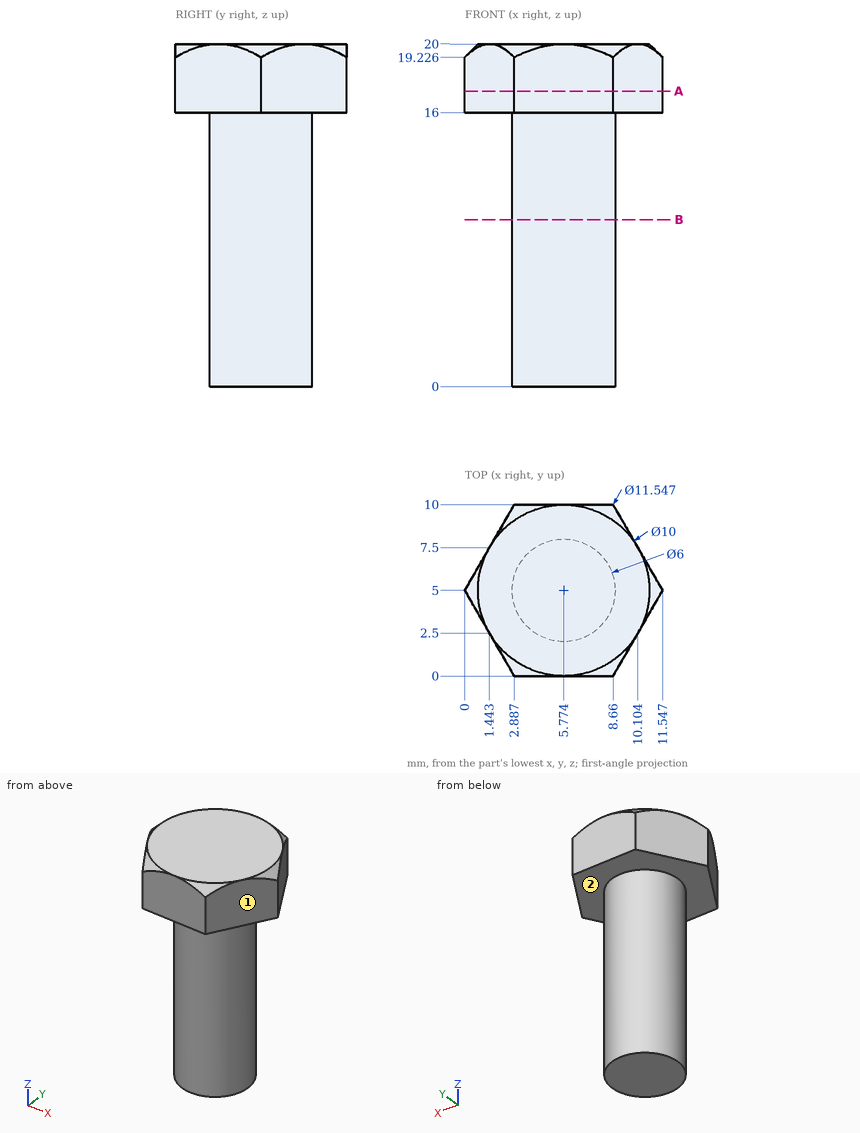
Here's the drawing with two shaded views (mm, measured from the low corner). I have some questions. A direction names the side the tool comes from. Coordinates: 2 decimals unless noted, no trailing zeros. Order: outer loops, then holes, each group sorted by start corner. A loop starts at its lowest first (then second) coordinate and runs counter-clockwise, first axis right, second up.
Q1. Suppose I cut it at B-B on z = 9.75. Please give me the cut outline in (x, y).
Q2. Suppose I cut it at A-A on z = 17.25. Please give me the cut outline in (x, y).
Q3. Will these pins go through, and if not, where does the flat tip stop? pin 1 (1 mm diameter, centred on x = 5.5, z = 4, fed in from +Y); pin 2 (6 mm diameter, centred on y = 1.5, z = 11.5, fed in from -X) (1 decimal); pin 3 (4 mm diameter, centred on y = 9, z = 16.5, fed in from +X).
Q4. Which directions (+Z, -Z, +X, -X, +Y, -Y) give clear straight access to the entire face, cutting with the end or side of a thin tool? Please do the marked faces 1 and 2.
Q5. Please list where these lines run through material, in increasing order: L1, parallel to Z at x = 1.5, y = 4.75; L2, parallel to X at y = 4.5, z = 2 (1 decimal); L3, parallel to Y at x = 5.25, z = 2.5 (1 decimal).
Answer:
1. outline: circle Ø6 at (5.77, 5)
2. outline: (0, 5) - (2.89, 0) - (8.66, 0) - (11.55, 5) - (8.66, 10) - (2.89, 10) - close
3. pin 1: stops at y = 8
3. pin 2: stops at x = 2.8
3. pin 3: stops at x = 10.39
4. face 1: +Z, -Z, +X, -Y
4. face 2: -Z
5. L1: z = 16 to 20
5. L2: x = 2.8 to 8.7
5. L3: y = 2 to 8
